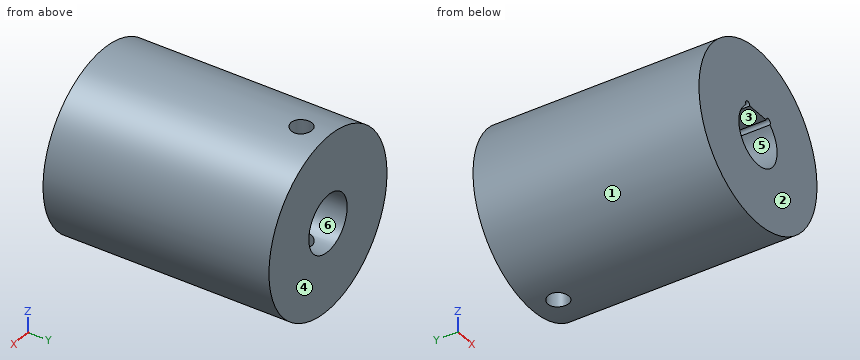
```python
from build123d import *

# Parameters (mm, degrees)
SKETCH1_R           = 7.257142857
BOSS_EXTRUDE1_DEPTH = 18.650857143
SKETCH2_R           = 2.358571483
CUT_EXTRUDE1_DEPTH  = 5.442857143
CUT_EXTRUDE2_DEPTH  = 10.16
SKETCH4_R           = 0.8636
CUT_EXTRUDE3_DEPTH  = 15.514285714
SCALE1_SCALE        = 1.75


with BuildPart() as part:
    # Sketch1 → Boss-Extrude1 (new body)
    with BuildSketch(Plane(origin=(0, 0, 0), x_dir=(1, 0, 0), z_dir=(0, 1, 0))):
        Circle(SKETCH1_R)
    extrude(amount=BOSS_EXTRUDE1_DEPTH)

    # Sketch2 → Cut-Extrude1 (cut)
    with BuildSketch(Plane(origin=(0, 18.650857143, 0), x_dir=(1, 0, 0), z_dir=(0, 1, 0))):
        Circle(SKETCH2_R)
    extrude(amount=-CUT_EXTRUDE1_DEPTH, mode=Mode.SUBTRACT)

    # Sketch3 → Cut-Extrude2 (cut)
    with BuildSketch(Plane.XZ):
        with BuildLine():
            Line((-1.008931831, 1.9812), (1.008931831, 1.9812))
            ThreePointArc((1.008931831, 1.9812), (1.340608786, 2.22303112), (1.469422309, 1.833288937))
            ThreePointArc((1.469422309, 1.833288937), (0, -2.3495), (-1.469422309, 1.833288937))
            ThreePointArc((-1.469422309, 1.833288937), (-1.340608786, 2.22303112), (-1.008931831, 1.9812))
        make_face()
    extrude(amount=-CUT_EXTRUDE2_DEPTH, mode=Mode.SUBTRACT)

    # Sketch4 → Cut-Extrude3 (cut, through all)
    with BuildSketch(Plane.XY.offset(7.257142857)):
        with Locations((0, 16.473714177)):
            Circle(SKETCH4_R)
    extrude(amount=-CUT_EXTRUDE3_DEPTH, mode=Mode.SUBTRACT)


with BuildPart() as part_1:
    # Scale1: scaled about (-4.09e-06, 9.303254996, 0.003077039)
    add(part.part.scale(SCALE1_SCALE).moved(Location((3.067e-06, -6.977441247, -0.002307779))))


solid = part_1.part
```
Geometry: final body of the model. Coordinates: model frame, mm. Face numbers are marked on the shaded views. A direction names the side the tool comes from. Coordinates: 2 decimals unless noted, no trailing zeros. Write each loop counter-clockwise with the first axis right and the second up, starting at its lowest first coordinate (ties: lowest second). Pieces come first, ordered by that corner, then holes. Notation, with made-up numbers: M 10.5,38.25 L 47.5,38.25 A11 cw 47.5,49.25 Z; hole C -38,14.25 d11. An arc over 180 degrees is marked long. Answer as CSV lines item,"result". Start each with the question number.
Q1. Reachability of the marked faces 4, 5 and 6 from +Z, -Z, +X, -X, +Y, -Y: full face, straight path, thin tool, end or side. Return the list, or none.
Q2. Cut plane B-B on z = 10.5. Return the cut outline in (x, y).
Q3. Cut plane C-C on y = -1.5. Return the cut outline in (x, z), then the cut area to 3 significant figures.
Q4. Line query: line 1 (Z direction, x = 3.5, y = -0.5); line 2 (X direction, y = 22, z = -7.75); line 3 (Z direction, x = 0, y = 2). Output: solid intervals per line, ascending. Write a range as from..to.
Q5. Cut plane D-D on z = -2.5. Return the cut outline in (x, y), then the cut area to 3 significant figures.
Q6. Pin query (flat end, axial travel): P1, Ø4, axis at x = -3.5, y = 1.5, coming from the +Z side; P2, Ø5, axis at x = 0, z = 0, coming from the -Y side; P3, Ø10, axis at y = 19, z = 9.5, coming from the -X side. Return the tip coordinate at first contact, or that it passes through.
Q7. Cut plane A-A on x = -1. Return the cut outline in (y, z), then the cut area to 3 significant figures.
Q8. Mould query, pull axis X, two halves, no side actions, for the marked faces 1, 2 and 3. Classes: released by +X, released by -X, zero draft, split by the parting line, or undercut.
Findings below:
1,face 4,"+Z, -Z, +X, -X, +Y"
1,face 5,"-Y"
1,face 6,"+Y"
2,outline,"M -7.14,-6.98 L 7.14,-6.98 L 7.14,25.66 L -7.14,25.66 Z; hole C 0,21.85 d3.02"
3,outline,"C 0,0 d25.4; hole M -2.57,3.21 A4.11 ccw long 2.57,3.21 A0.44 ccw long 1.77,3.46 L -1.77,3.46 A0.44 ccw long Z"
3,area,"455 mm2"
4,line 1,"z = -12.21..-2.16, 2.16..12.21"
4,line 2,"x = -10.06..-1.5, 1.5..10.06"
4,line 3,"z = -12.7..-4.11, 3.46..12.7"
5,outline,"M -12.45,-6.98 L -3.27,-6.98 L -3.27,10.8 L 3.27,10.8 L 3.27,-6.98 L 12.45,-6.98 L 12.45,25.66 L 3.29,25.66 L 3.29,16.14 L -3.29,16.14 L -3.29,25.66 L -12.45,25.66 Z"
5,area,"634 mm2"
6,P1,"stops at z = 12.61"
6,P2,"stops at y = 10.8"
6,P3,"stops at x = -11.88"
7,outline,"M -6.98,-12.66 L 20.72,-12.66 L 20.72,-4.01 L 16.14,-4.01 L 16.14,4 L 20.72,4 L 20.72,12.66 L -6.98,12.66 L -6.98,3.46 L 10.8,3.46 L 10.8,-3.99 L -6.98,-3.99 Z; M 22.98,-12.66 L 25.66,-12.66 L 25.66,-4.01 L 22.98,-4.01 Z; M 22.98,4 L 25.66,4 L 25.66,12.66 L 22.98,12.66 Z"
7,area,"578 mm2"
8,face 1,"split by the parting line"
8,face 2,"zero draft"
8,face 3,"undercut"
